Read the model definition and answer for the solid it produces. Units are mm, in the model's axes. Face numbers are marked on the shaded views. A direction names the side the tool comes from. Coordinates: 2 decimals unless noted, no trailing zeros. Write each loop counter-clockwise with the first axis right and the second up, starting at its lowest first coordinate (ties: lowest second). Pieces come first, ordered by that corner, then holes. Notation, with made-up numbers: (31.25, 30.5) -> (72.25, 30.5) arc R18 cw to (72.25, 47.5) -> close; hole circle Ø11 at (56.25, -3). An arc over 180 degrees is marked (long way). Return JSON: item names as keys, results as strings.
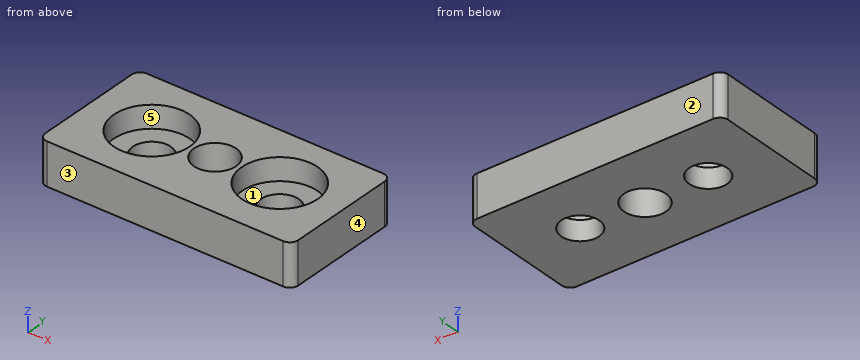
from build123d import *

# Parameters (mm, degrees)
SKETCH1_W                               = 60
SKETCH1_H                               = 30
BOSS_EXTRUDE1_DEPTH                     = 10
F_10_0_10_DIAMETER_HOLE1_D              = 10
CBORE_FOR_M8_HEX_HEAD_BOLT1_D           = 9
CBORE_FOR_M8_HEX_HEAD_BOLT1_CBORE_D     = 18.011
CBORE_FOR_M8_HEX_HEAD_BOLT1_CBORE_DEPTH = 5.3
FILLET1_R                               = 2


with BuildPart() as part:
    # Sketch1 → Boss-Extrude1 (new body)
    with BuildSketch(Plane.XY.offset(10)):
        Rectangle(SKETCH1_W, SKETCH1_H)
    extrude(amount=-BOSS_EXTRUDE1_DEPTH)

    # Ø10.0 (10) Diameter Hole1 (through all)
    with Locations(Plane.XY.offset(10)):
        with Locations((0, 0)):
            Hole(F_10_0_10_DIAMETER_HOLE1_D / 2)

    # CBORE for M8 Hex Head Bolt1 (through all)
    with Locations(Plane.XY.offset(10)):
        with Locations((-15, 0), (15, 0.462807071)):
            CounterBoreHole(CBORE_FOR_M8_HEX_HEAD_BOLT1_D / 2, CBORE_FOR_M8_HEX_HEAD_BOLT1_CBORE_D / 2, CBORE_FOR_M8_HEX_HEAD_BOLT1_CBORE_DEPTH)

    # Fillet1
    fillet1_edges = [part.edges().sort_by_distance(p)[0] for p in [
        (30, -15, 5),
        (-30, -15, 5),
        (-30, 15, 5),
        (30, 15, 5),
    ]]
    fillet(fillet1_edges, radius=FILLET1_R)


solid = part.part
1. For a pull along Y with two mould halves and no side action, classify the marked faces 3, 4 and 5 as +Y half, -Y half, draft (parallel to the pull), parting line (faces both ways), or undercut.
Taken from the geometry:
{"face 3": "-Y half", "face 4": "draft", "face 5": "undercut"}
2. The part is cut by section A-A (x = -15). Determine the outline of the cut face in (y, z).
Taken from the geometry:
{"outline": "(-15, 0) -> (-4.5, 0) -> (-4.5, 4.7) -> (-9.01, 4.7) -> (-9.01, 10) -> (-15, 10) -> close; (4.5, 0) -> (15, 0) -> (15, 10) -> (9.01, 10) -> (9.01, 4.7) -> (4.5, 4.7) -> close"}
3. The part is cut by section B-B (z = 2.25). Determine the outline of the cut face in (x, y).
Taken from the geometry:
{"outline": "(-30, -13) arc R2 ccw to (-28, -15) -> (28, -15) arc R2 ccw to (30, -13) -> (30, 13) arc R2 ccw to (28, 15) -> (-28, 15) arc R2 ccw to (-30, 13) -> close; hole circle Ø9 at (-15, 0); hole circle Ø10 at (0, 0); hole circle Ø9 at (15, 0.46)"}
4. A tool of negligible diameter and unlimited length cuts with its end or side. For the marked faces 1 and 2, from which of +Z, -Z, +X, -X, +Y, -Y can it reach the whole face along a straight path? Write none if from no direction.
Taken from the geometry:
{"face 1": "+Z", "face 2": "+Z, -Z, +X, -X, +Y"}
5. Flat-ended cylindrical pins translate along their axes: pin 1 Ø10.5 at (x, y) = (-15, 0) entering from +Z; pin 2 Ø10 at (x, y) = (18.5, 9.5) entering from -Z. Find the tip coordinate at first contact, or state that the pin passes through.
Taken from the geometry:
{"pin 1": "stops at z = 4.7", "pin 2": "stops at z = 0"}
6. Consider L1, parallel to Y at x = -15, z = 2.75; L2, parallel to X at y = 2, z = 6.75; L3, parallel to Y at x = 15, z = 1. Determine where each line is inside the solid, lowest interval first.
Taken from the geometry:
{"L1": "y = -15 to -4.5, 4.5 to 15", "L2": "x = -30 to -23.78, -6.22 to -4.58, 4.58 to 6.13, 23.87 to 30", "L3": "y = -15 to -4.04, 4.96 to 15"}
7. The part is cut by section C-C (y = 6.25). Determine the outline of the cut face in (x, z), then the cut area to 3 significant figures.
Taken from the geometry:
{"outline": "(-30, 0) -> (30, 0) -> (30, 10) -> (21.9, 10) -> (21.9, 4.7) -> (8.1, 4.7) -> (8.1, 10) -> (-8.52, 10) -> (-8.52, 4.7) -> (-21.48, 4.7) -> (-21.48, 10) -> (-30, 10) -> close", "area": "458 mm2"}
8. The part is cut by section D-D (x = 0). Determine the outline of the cut face in (y, z).
Taken from the geometry:
{"outline": "(-15, 0) -> (-5, 0) -> (-5, 10) -> (-15, 10) -> close; (5, 0) -> (15, 0) -> (15, 10) -> (5, 10) -> close"}
